Drawing for the job (mm, zero at the part's lowest x, y, z). A direction names the side the tool comes from. Round coordinates to 2 decimals unless told otherwise and drop trailing zeros. Write each loop counter-clockwise with the first axis right and the second up, starting at its lowest first coordinate (ties: lowest second). Pieces come first, ordered by that corner, then holes. Notation, with made-up numbers: M 6,75 L 63,75 A6 ccw 63,79 Z; hole C -15,78.25 d2. An arc over 180 degrees is marked long. Use a Markdown table: item, result.
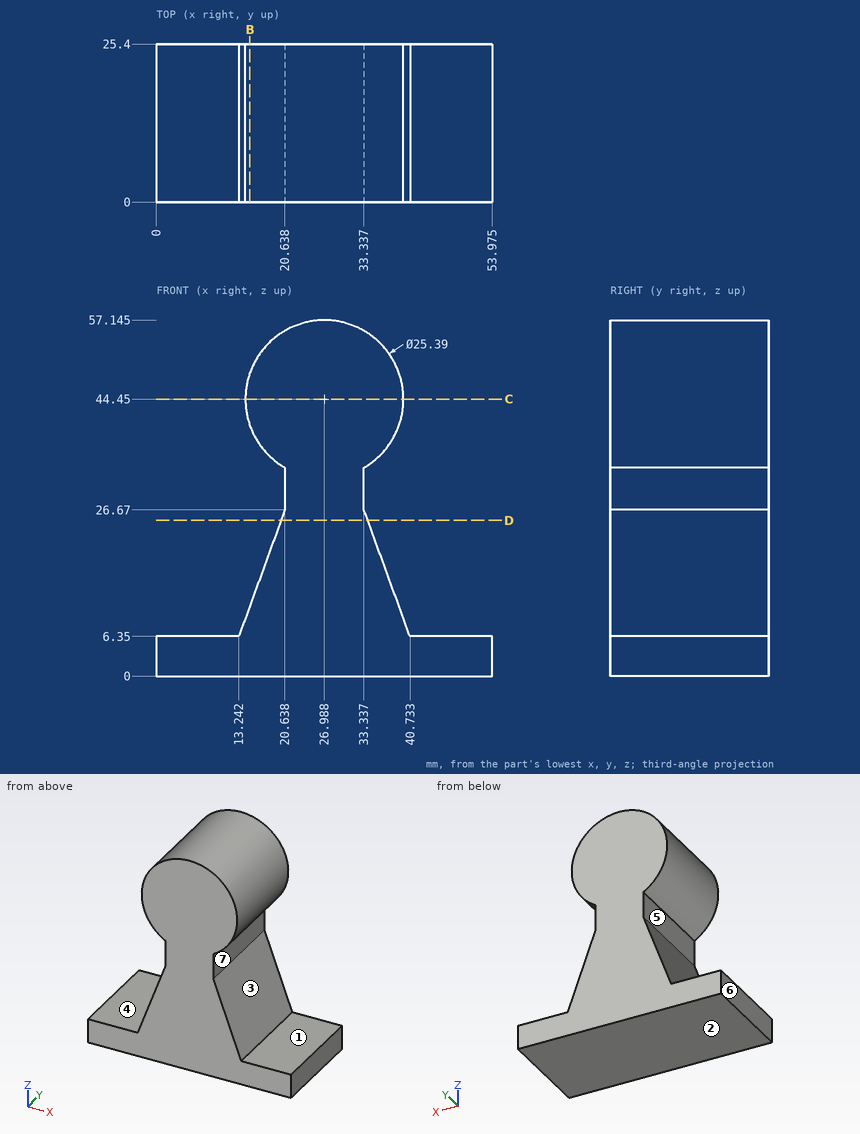
Q1. Cut at C-C on z = 44.45. Give the cut face in (x, y), and give its area (3 significant figures).
Response values:
| item | result |
|---|---|
| outline | M 14.29,0 L 39.68,0 L 39.68,25.4 L 14.29,25.4 Z |
| area | 645 mm2 |
Q2. Cut at D-D on z = 25. Give the cut face in (x, y) (1 decimal).
Response values:
| item | result |
|---|---|
| outline | M 20,0 L 33.9,0 L 33.9,25.4 L 20,25.4 Z |
Q3. Which spindle directions (+Z, -Z, +X, -X, +Y, -Y) get a long thin tool onto all of the face, cutting with end or side? Do the marked faces 4, 5, 6 and 7. Say none if no direction does.
Response values:
| item | result |
|---|---|
| face 4 | +Z, -X, +Y, -Y |
| face 5 | -X, +Y, -Y |
| face 6 | +Z, -Z, -X, +Y, -Y |
| face 7 | +X, +Y, -Y |
Q4. Cut at B-B on x = 15. Give the cut face in (y, z), and give its area (3 significant figures).
Response values:
| item | result |
|---|---|
| outline | M 0,0 L 25.4,0 L 25.4,11.18 L 0,11.18 Z; M 0,40.27 L 25.4,40.27 L 25.4,48.63 L 0,48.63 Z |
| area | 496 mm2 |
Q5. Two-plate mould, pull along Z, no slides. Class the marked faces 1, 2 and 3: +Z half, -Z half, draft (parallel to the pull), parting line (faces both ways), or undercut.
Response values:
| item | result |
|---|---|
| face 1 | +Z half |
| face 2 | -Z half |
| face 3 | undercut |
Q6. Drop flat-ended pins along their axis: P1, Ø3.5, axis at y = 7.5, z = 30, coming from the +X side; P2, Ø10, axis at y = 21, z = 14.5, coming from the +X side; P3, Ø1.5, axis at y = 18.5, z = 26.5, coming from the -X side; P4, Ø4, axis at x = 21.5, z = 43, coming from the -Y side. Give the stop position or say it passes through.
Response values:
| item | result |
|---|---|
| P1 | stops at x = 33.34 |
| P2 | stops at x = 39.59 |
| P3 | stops at x = 20.3 |
| P4 | stops at y = 0 |
Q7. Drill centre lines: L1, parallel to X at y = 9.5, z = 33; L2, parallel to Z at x = 44, y = 15.25; L3, parallel to Z at x = 21, y = 14.75 (1 decimal). Where is each one in solid material? Low to high.
Response values:
| item | result |
|---|---|
| L1 | x = 20.64 to 33.34 |
| L2 | z = 0 to 6.35 |
| L3 | z = 0 to 55.6 |
